Autodesk Fusion 360 part; units mm, degrees
sketch "Sketch1" plane through (0, 0, 0) normal (0, 1, 0) x (1, 0, 0)
  line L0 (0, 0) -> (185, 0)
  line L1 (185, 0) -> (185, -79)
  line L2 (185, -79) -> (0, -79)
  line L3 (0, -79) -> (0, 0)
extrude "Extrude1" add sketch "Sketch1" along normal blind 2
sketch "Sketch2" plane through (0, 0, 0) normal (0, 1, 0) x (1, 0, 0)
  line L0 (11, -24) -> (28, -24)
  line L1 (28, -24) -> (28, -55)
  line L2 (28, -55) -> (11, -55)
  line L3 (11, -55) -> (11, -24)
extrude "Extrude2" cut sketch "Sketch2" along normal blind 5
fillet "Fillet1" radius 1 1 edges at (185, 1, 79)
fillet "Fillet2" radius 1 1 edges at (185, 1, 0)
fillet "Fillet3" radius 1 1 edges at (0, 1, 79)
fillet "Fillet4" radius 1 1 edges at (0, 1, 0)
fillet "Fillet5" radius 1 1 edges at (28, 1, 55)
fillet "Fillet6" radius 1 1 edges at (11, 1, 55)
fillet "Fillet7" radius 1 1 edges at (11, 1, 24)
fillet "Fillet8" radius 1 1 edges at (28, 1, 24)
Geometry: final body of the model. Coordinates: model frame, mm. Give positions to 0.01 mm unless a question says otherwise; leave off trailing zeros. Write each loop counter-clockwise with the first axis right and the second up, starting at its lowest first coordinate (ties: lowest second). Pieces come first, ordered by that corner, then holes. Notation, with made-up numbers: (-18, -9) - (22, -9) arc R15 cw to (22, 18) - close; hole circle Ø9 at (-24, 16). An arc over 180 degrees is marked (long way). Return JSON: item names as keys, results as strings. Group by question number.
1) Section A-A on y = 0.7. Return the cut outline in (x, z).
2) Line query: line 1 (X direction, y = 0.9, z = 51); line 2 (Z direction, x = 17, y = 1.8). Output: solid intervals per line, ascending.
3) First-contact query: P1, Ø0.6, axis at y = 1, z = 34, coming from the -X side. Flat tip, straight axial feed; report the tip coordinate or a pass-through.
4) Section B-B on z = 47. Return the cut outline in (x, y).
Filled in:
{
 "1": {"outline": "(0, 1) arc R1 ccw to (1, 0) - (184, 0) arc R1 ccw to (185, 1) - (185, 78) arc R1 ccw to (184, 79) - (1, 79) arc R1 ccw to (0, 78) - close; hole (11, 25) arc R1 ccw to (12, 24) - (27, 24) arc R1 ccw to (28, 25) - (28, 54) arc R1 ccw to (27, 55) - (12, 55) arc R1 ccw to (11, 54) - close"},
 "2": {"line 1": "x = 0 to 11, 28 to 185", "line 2": "z = 0 to 24, 55 to 79"},
 "3": {"P1": "stops at x = 0"},
 "4": {"outline": "(0, 0) - (11, 0) - (11, 2) - (0, 2) - close; (28, 0) - (185, 0) - (185, 2) - (28, 2) - close"}
}
